Autodesk Inventor part; units mm, degrees
ref_plane "YZ Plane" through (0, 0, 0) normal (1, 0, 0) x (0, 1, 0)
ref_plane "XZ Plane" through (0, 0, 0) normal (0, 1, 0) x (-1, 0, 0)
ref_plane "XY Plane" through (0, 0, 0) normal (0, 0, 1) x (1, 0, 0)
sketch "Sketch1" plane through (0, 0, 0) normal (0, 1, 0) x (-1, 0, 0)
  point P0 (0, 0)
sketch "Sketch2" plane through (0, 0, 0) normal (0, 1, 0) x (-1, 0, 0)
  line L0 (0, -25) -> (0, -30)
  line L1 (0, -30) -> (1.5, -30)
  line L2 (1.5, -30) -> (1.5, -25.8289)
  line L3 (1.5, -25.8289) -> (23.5, -12)
  line L4 (23.5, -12) -> (23.5, -4.75)
  line L5 (23.5, -4.75) -> (22, -4.75)
  line L6 (22, -4.75) -> (22, -11.1711)
  line L7 (22, -11.1711) -> (0, -25)
  line L8 (28.2, 0) -> (-4.7, 0)
  line L9 (0, -36) -> (0, 6)
  dimension "d6" = 1.5
  dimension "d7" = 1.5
  dimension "d8" = 4.75
  dimension "d9" = 7.25
  dimension "d10" = 5
  dimension "d11" = 30
  dimension "d12" = 23.5
  dimension "d13" = 1.5
revolve "Revolution1" add sketch "Sketch2" angle 360 about axis through (-10, 0, 0) along (1, 0, 0)
properties part number "base-biotrap"
CAD build for the part. Positions are in the model's coordinates, mm. A direction names the side the tool comes from. Coordinates: 2 decimals unless noted, no trailing zeros. Loops run counter-clockwise (first coordinate to the right, second up) from the corner with the lowest first, then second, coordinate; pieces in that order, holes last. Notation, with made-up numbers: (4, 26.25) - (46, 26.25) arc R27 ccw to (46, 50.25) - close; hole circle Ø8 at (-34, 42). An arc over 180 degrees is marked (long way). Return JSON: item names as keys, results as strings.
1. 3-axis set-ups, long thin cutter, end or side, ignore diameter. For faces 1 (the flat face through (0, 25, 7)), 2 (the flat face through (-22, 0, -5)), 3 (the flat face through (-1.5, 22.4, -13.2)): which of +Z, -Z, +X, -X, +Y, -Y reach the whole face in a straight line?
Result:
{"face 1": "+Z, -Z, +X, +Y, -Y", "face 2": "+X", "face 3": "-X"}
2. Band-saw the part on A-A (z = 0). Give the cut face in (x, y), and give its area (3 significant figures).
Result:
{"outline": "(-23.5, -12) - (-1.5, -25.83) - (-1.5, -30) - (0, -30) - (0, -25) - (-22, -11.17) - (-22, -4.75) - (-23.5, -4.75) - close; (-23.5, 4.75) - (-22, 4.75) - (-22, 11.17) - (0, 25) - (0, 30) - (-1.5, 30) - (-1.5, 25.83) - (-23.5, 12) - close", "area": "112 mm2"}
3. Mould opens along Y. For faces 4 (the conical face through (-22.124, 3.864, -12.271)), 5 (the flat face through (-23.5, 0, -5)), 6 (the cylindrical face through (-22.74, -4.214, -2.192)) say: released by +Y, released by -Y, zero draft, split by the parting line, or undercut.
Result:
{"face 4": "split by the parting line", "face 5": "zero draft", "face 6": "undercut"}
4. Drop flat-ended pins along their axis: pin 1 (6.5 mm diameter, centred on y = 0, z = 2.5, fed in from +X); pin 2 (1 mm diameter, centred on x = -14, z = 15, fed in from -Y); pin 3 (8.5 mm diameter, centred on y = 0, z = 0, fed in from -X); pin 4 (6 mm diameter, centred on x = -14.5, y = -9.5, fed in from -Z). Give the stop position or say it passes through.
Result:
{"pin 1": "stops at x = -22", "pin 2": "stops at y = -10.8", "pin 3": "passes through", "pin 4": "stops at z = -17.56"}
5. Band-saw the part on D-D (x = -16.5). Give the cut face in (y, z), and give its area (3 significant figures).
Result:
{"outline": "circle Ø32.8 at (0, 0); hole circle Ø29.26 at (0, 0)", "area": "173 mm2"}
6. Band-saw the part on C-C (x = -12.25). Give the cut face in (y, z), and give its area (3 significant figures).
Result:
{"outline": "circle Ø38.14 at (0, 0); hole circle Ø34.6 at (0, 0)", "area": "202 mm2"}
7. Probe L1, parallel to Y at x = -22.85, z = 0; L2, parallel to Y at x = -22.6, z = 0; L3, parallel to Z at x = -10.25, y = -8.5. List the from-to ranges inside material, lowest first. Write a range as from..to.
Result:
{"L1": "y = -12.41..-4.75, 4.75..12.41", "L2": "y = -12.57..-4.75, 4.75..12.57", "L3": "z = -18.47..-16.5, 16.5..18.47"}
